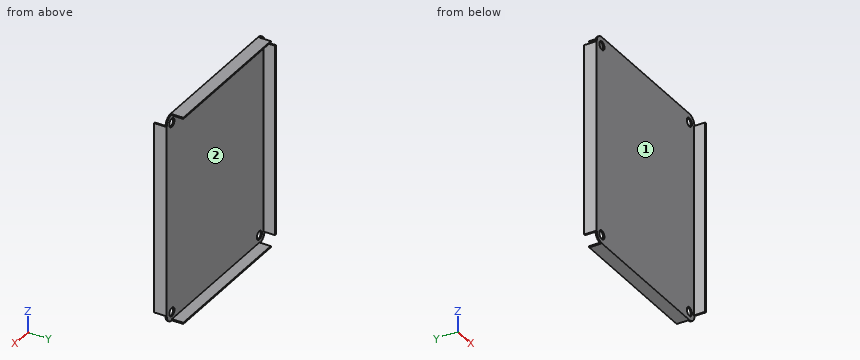
Autodesk Inventor part; units mm, degrees
ref_plane "YZ Plane" through (0, 0, 0) normal (1, 0, 0) x (0, 1, 0)
ref_plane "XZ Plane" through (0, 0, 0) normal (0, 1, 0) x (-1, 0, 0)
ref_plane "XY Plane" through (0, 0, 0) normal (0, 0, 1) x (1, 0, 0)
sketch "Sketch1" plane through (0, 0, 0) normal (0, 1, 0) x (-1, 0, 0)
  line L0 (0, 0) -> (-361.95, 0)
  line L1 (-361.95, 0) -> (-361.95, -463.55)
  line L2 (-361.95, -463.55) -> (0, -463.55)
  line L3 (0, -463.55) -> (0, 0)
  dimension "d0" = 361.95
  dimension "d1" = 463.55
extrude "Extrusion1" add sketch "Sketch1" along normal blind 2.794
fillet "Fillet1" radius 19.05 4 edges at (361.95, 1.397, 0) (361.95, 1.397, -463.55) (0, 1.397, -463.55) (0, 1.397, 0)
sketch "Sketch3" plane through (0, 0, 0) normal (0, -1, 0) x (1, 0, 0)
  line L0 (361.95, -19.05) -> (359.3341, -19.05)
  line L1 (359.3341, -19.05) -> (359.3341, -444.5)
  line L2 (359.3341, -444.5) -> (361.95, -444.5)
  line L3 (361.95, -444.5) -> (361.95, -19.05)
  point P0 (0, 0)
extrude "Extrusion2" add sketch "Sketch3" along normal blind 25.4
sketch "Sketch4" plane through (0, 2.794, 0) normal (0, 1, 0) x (1, 0, 0)
  line L0 (19.05, 0) -> (342.8936, 0)
  line L1 (342.8936, 0) -> (342.8936, 2.7101)
  line L2 (342.8936, 2.7101) -> (19.05, 2.7101)
  line L3 (19.05, 2.7101) -> (19.05, 0)
  line L4 (0, 19.05) -> (2.9466, 19.05)
  line L5 (2.9466, 19.05) -> (2.9466, 444.7516)
  line L6 (2.9466, 444.7516) -> (0, 444.7516)
  line L7 (0, 444.7516) -> (0, 19.05)
  line L8 (342.9, 463.55) -> (19.05, 463.55)
  line L9 (19.05, 463.55) -> (19.05, 460.6098)
  line L10 (19.05, 460.6098) -> (342.9, 460.6098)
  line L11 (342.9, 460.6098) -> (342.9, 463.55)
  point P0 (0, 0)
extrude "Extrusion3" add sketch "Sketch4" along normal blind 25.4
sketch "Sketch5" plane through (0, 2.794, 0) normal (0, 1, 0) x (1, 0, 0)
  line L0 (19.05, 460.6098) -> (19.05, 463.55)
  arc A0 (19.05, 463.55) -> (0.0017, 444.7516) centre (19.05, 444.5) ccw
  line L1 (0.0017, 444.7516) -> (2.9466, 444.7516)
  line L2 (2.9466, 444.7516) -> (2.9466, 19.05)
  line L3 (2.9466, 19.05) -> (0, 19.05)
  arc A1 (0, 19.05) -> (19.05, 0) centre (19.05, 19.05) ccw
  line L4 (19.05, 0) -> (19.05, 2.7101)
  line L5 (19.05, 2.7101) -> (342.8936, 2.7101)
  line L6 (342.8936, 2.7101) -> (342.8936, 0)
  line L7 (342.8936, 0) -> (342.9, 0)
  arc A2 (342.9, 0) -> (361.95, 19.05) centre (342.9, 19.05) ccw
  line L8 (361.95, 19.05) -> (361.95, 444.5)
  arc A3 (361.95, 444.5) -> (342.9, 463.55) centre (342.9, 444.5) ccw
  line L9 (342.9, 463.55) -> (342.9, 460.6098)
  line L10 (342.9, 460.6098) -> (19.05, 460.6098)
  circle A4 centre (19.05, 19.05) radius 9.525
  circle A5 centre (19.05, 444.5) radius 9.525
  point P0 (0, 0)
  dimension "d11" = 19.05
  dimension "d12" = 19.05
extrude "Extrusion4" cut sketch "Sketch5" against normal blind 25.4 contours A4 | A5
sketch "Sketch6" plane through (0, 2.794, 0) normal (0, 1, 0) x (1, 0, 0)
  circle A0 centre (19.05, 19.05) radius 9.525
  circle A1 centre (19.05, 444.5) radius 9.525
  line L0 (19.05, 460.6098) -> (19.05, 463.55)
  arc A2 (19.05, 463.55) -> (0.0017, 444.7516) centre (19.05, 444.5) ccw
  line L1 (0.0017, 444.7516) -> (2.9466, 444.7516)
  line L2 (2.9466, 444.7516) -> (2.9466, 19.05)
  line L3 (2.9466, 19.05) -> (0, 19.05)
  arc A3 (0, 19.05) -> (19.05, 0) centre (19.05, 19.05) ccw
  line L4 (19.05, 0) -> (19.05, 2.7101)
  line L5 (19.05, 2.7101) -> (342.8936, 2.7101)
  line L6 (342.8936, 2.7101) -> (342.8936, 0)
  line L7 (342.8936, 0) -> (342.9, 0)
  arc A4 (342.9, 0) -> (361.95, 19.05) centre (342.9, 19.05) ccw
  line L8 (361.95, 19.05) -> (361.95, 444.5)
  arc A5 (361.95, 444.5) -> (342.9, 463.55) centre (342.9, 444.5) ccw
  line L9 (342.9, 463.55) -> (342.9, 460.6098)
  line L10 (342.9, 460.6098) -> (19.05, 460.6098)
  circle A6 centre (342.9, 19.05) radius 9.525
  circle A7 centre (342.9, 444.5) radius 9.525
  point P0 (0, 0)
  dimension "d15" = 19.05
  dimension "d16" = 19.05
extrude "Extrusion5" cut sketch "Sketch6" against normal blind 25.4 contours A6 | A7
properties part number "Cart_MID_SHELF"
The listing builds one solid part. Answer for the finished solid, in the listing's coordinates (mm). Face numbers are marked on the shaded views. Round coordinates to 2 decimals unless told otherwise and drop trailing zeros. Order: outer loops, then holes, each group sorted by start corner. A loop starts at its lowest first (then second) coordinate and runs counter-clockwise, first axis right, second up. Notation, with made-up numbers: M 76.25,-25 L 81.25,-25 A32 cw 81.25,6 Z; hole C 39.5,5 d7. An arc over 180 degrees is marked long. Answer in a Markdown table with one row per item. Add a question column.
1) The part is cut by section A-A on x = 84. Determine the outline of the cut face in (y, z), plus the area to 3 significant figures.
2) Flat-ended cylindrical pins translate along their axes: pin 1 Ø11.5 at (x, z) = (342.9, -19.05) entering from +Y; pin 2 Ø1.5 at (y, z) = (18.5, -335) entering from +X; pin 3 Ø12 at (x, z) = (311, -49.5) entering from +Y; pin 4 Ø3 at (y, z) = (11, -463) entering from +X. Find the tip coordinate at first contact, or state that the pin passes through.
3) The part is cut by section B-B on z = -368. Determine the outline of the cut face in (x, y).
4) The part is cut by section C-C on y = -16. Determine the outline of the cut face in (x, z), plus the area to 3 significant figures.
5) Consider line 1 along X through (y, z) = (1.15, -19.05) (3 decimals); line 2 along Z through (x, y) = (19.05, 1.3) (3 decimals). Determine where each line is inside the solid, lowest interval first. Write a range as from..to.
6) Determine the mould class of the marked faces 1 and 2 for opening direction Z: pulls with the +Z half, pulls with the -Z half, needs draft (parallel to the pull), parting line crosses it, or undercut.
Findings below:
| question | item | result |
|---|---|---|
| 1 | outline | M 0,-463.55 L 28.19,-463.55 L 28.19,-460.61 L 2.79,-460.61 L 2.79,-2.71 L 28.19,-2.71 L 28.19,0 L 0,0 Z |
| 1 | area | 1,440 mm² |
| 2 | pin 1 | passes through |
| 2 | pin 2 | stops at x = 2.95 |
| 2 | pin 3 | stops at y = 2.79 |
| 2 | pin 4 | stops at x = 342.9 |
| 3 | outline | M 0,0 L 359.33,0 L 359.33,-25.4 L 361.95,-25.4 L 361.95,2.79 L 2.95,2.79 L 2.95,28.19 L 0,28.19 Z |
| 4 | outline | M 359.33,-444.5 L 361.95,-444.5 L 361.95,-19.05 L 359.33,-19.05 Z |
| 4 | area | 1,110 mm² |
| 5 | line 1 | x = 0..9.525, 28.575..333.375, 352.425..361.95 |
| 5 | line 2 | z = -463.55..-454.025, -434.975..-28.575, -9.525..0 |
| 6 | face 1 | needs draft |
| 6 | face 2 | undercut |
